Geometry: see drawing. Coordinates: mm, zero at the bounding-box minimum. A direction names the side the tool comes from. Round coordinates to 2 decimals unless told otherwise and drop trailing zeros. Write each loop counter-clockwise with the first axis right and the second up, starting at its lowest first coordinate (ties: lowest second). Pieces come first, ordered by that corner, then holes. Notation, with made-up numbers: M -15.5,82.5 L -1.5,82.5 A27 cw -1.5,121.5 Z; hole C 49,59.25 d11. An arc over 180 degrees is marked long. Use one line per item in the form item = value. Start each with the question number.
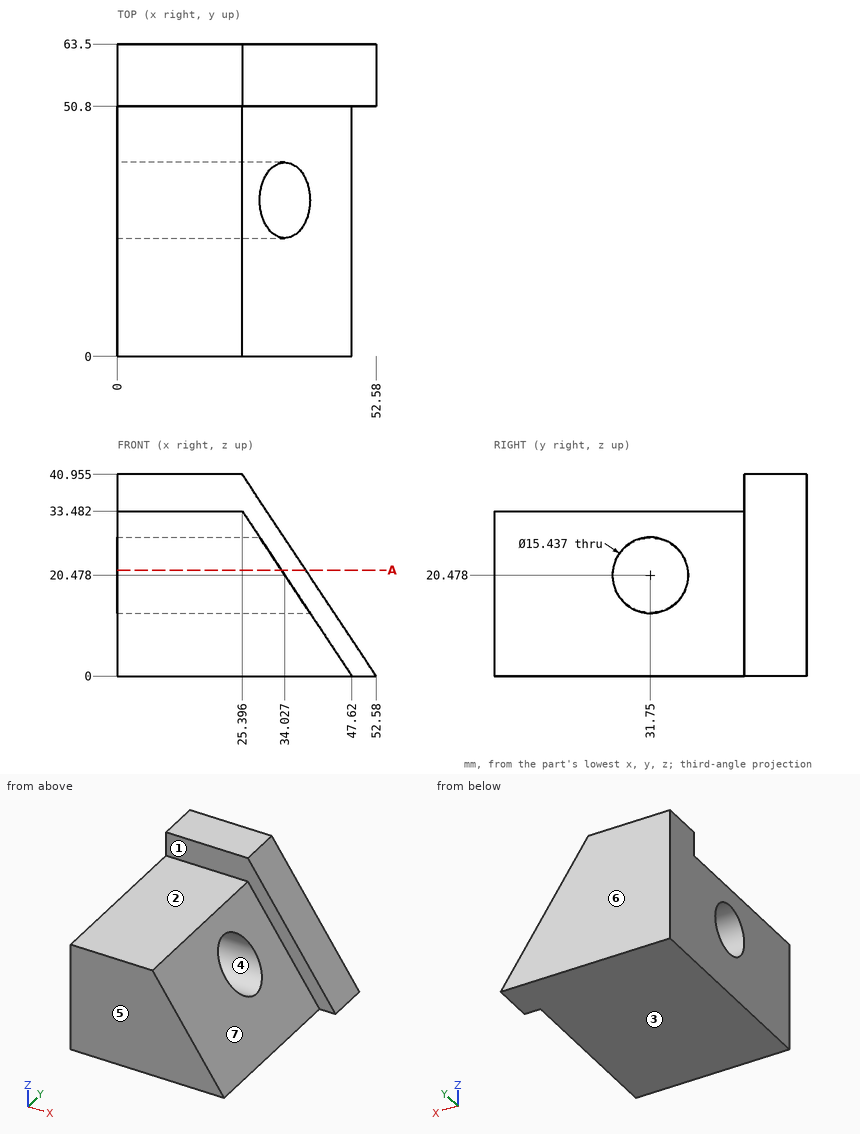
Item 1: Cut plane A-A (z = 21.5). Output: boundary loops of the cut face in (x, y).
Item 2: Draft query along Y for the marked faces 4, 5, 6 and 7. Return one class per face: +Y half, -Y half, draft (parallel to the pull), parting line (faces both ways), or undercut.
Item 3: Ray query, line 1 (Z direction, x = 8, y = 31.75); line 2 (Y direction, x = 21, z = 21); line 3 (Y direction, x = 22.5, z = 17). Return the intervals inside material, ascending. Write a range as from..to.
Item 4: First-contact query: pin 1 (18 mm diameter, centred on y = 31.75, z = 20.48, fed in from +X); pin 2 (2 mm diameter, centred on x = 32.5, y = 23.5, fed in from +Z) (1 decimal); pin 3 (3 mm diameter, centred on x = 36.5, y = 26, fed in from +Z) (1 decimal). Flat tips, straight axial feed; report the tip coordinate or a pass-through.
Item 5: Reachability of the marked faces 1, 2 and 3 from +Z, -Z, +X, -X, +Y, -Y: full face, straight path, thin tool, end or side. Return the list, or none.
Final values:
q1.outline = M 0,0 L 33.35,0 L 33.35,24.1 L 0,24.1 Z; M 0,39.4 L 33.35,39.4 L 33.35,50.8 L 38.31,50.8 L 38.31,63.5 L 0,63.5 Z
q2.face_4 = undercut
q2.face_5 = -Y half
q2.face_6 = +Y half
q2.face_7 = draft
q3.line_1 = 0..12.76, 28.2..33.48
q3.line_2 = 0..24.05, 39.45..63.5
q3.line_3 = 0..24.86, 38.64..63.5
q4.pin_1 = 40
q4.pin_2 = 24.3
q4.pin_3 = 17.6
q5.face_1 = +Z, +X, -Y
q5.face_2 = +Z, +X, -X, -Y
q5.face_3 = -Z, +X, -X, +Y, -Y
